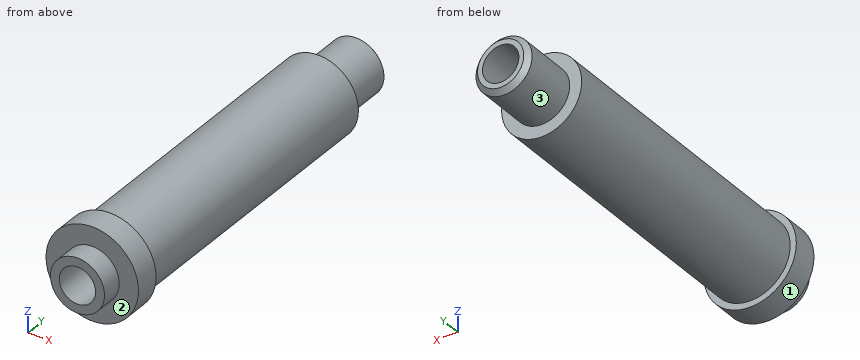
Autodesk Inventor part; units mm, degrees
ref_plane "YZ Plane" through (0, 0, 0) normal (1, 0, 0) x (0, 1, 0)
ref_plane "XZ Plane" through (0, 0, 0) normal (0, 1, 0) x (-1, 0, 0)
ref_plane "XY Plane" through (0, 0, 0) normal (0, 0, 1) x (1, 0, 0)
sketch "Sketch1" plane through (0, 0, 0) normal (0, 1, 0) x (-1, 0, 0)
  circle A0 centre (0, 0) radius 4.699
  dimension "d0" = 9.398
extrude "Extrusion1" add sketch "Sketch1" along normal blind 4.826
sketch "Sketch2" plane through (0, 0, 0) normal (0, -1, 0) x (1, 0, 0)
  circle A0 centre (0, 0) radius 4.075
  dimension "d3" = 8.15
extrude "Extrusion2" add sketch "Sketch2" against normal blind 35.866
sketch "Sketch3" plane through (0, 0, 0) normal (0, -1, 0) x (1, 0, 0)
  circle A0 centre (0, 0) radius 4.699
  circle A1 centre (0, 0) radius 2.75
  dimension "d18" = 5.5
extrude "Extrusion3" cut sketch "Sketch3" against normal blind 2.2
sketch "Sketch5" plane through (0, 0, 0) normal (0, -1, 0) x (1, 0, 0)
  circle A0 centre (0, 0) radius 2.75
hole "Hole2" at (0, 0, 0) direction (0, 1, 0) diameter 3.7 end through all
sketch "Sketch6" plane through (0, 35.866, 0) normal (0, 1, 0) x (1, 0, 0)
  circle A0 centre (0, 0) radius 1.85
  circle A1 centre (0, 0) radius 2.85
  dimension "d29" = 5.7
extrude "Extrusion4" add sketch "Sketch6" along normal blind 6.1
chamfer "Chamfer3" distance 0.5 angle 45 1 edges at (-2.85, 41.966, 0)
properties part number "Hour shaft test 7"
Geometry check sheet. Reference: the model listing, model coordinates, mm. Face numbers are marked on the shaded views. A direction names the side the tool comes from. Round coordinates to 2 decimals unless told otherwise and drop trailing zeros. Order: outer loops, then holes, each group sorted by start corner. A loop starts at its lowest first (then second) coordinate and runs counter-clockwise, first axis right, second up. Notation, with made-up numbers: (51.25, 89) - (79.25, 89) arc R18 ccw to (79.25, 111) - close; hole circle Ø8 at (-30, -16.75). An arc over 180 degrees is marked (long way). Use a Markdown table: item, result. Add a question column.
(1) Sectioned sample at A-A, the plane x = 0. Enter the section's corners in (y, z) (3 decimals), and give its area (3 significant figures).
(2) Sectioned sample at B-B, the plane z = 0. Enter the section's corners in (x, y) (3 decimals).
(3) Tool access check on the marked faces 1, 2 and 3. Record the directions out of +Z, -Z, +X, -X, +Y, -Y that give a thin tool (end or side, any length) a straight path to the whole face; none if there is none.
(4) Sectioned sample at D-D, the plane x = -3.5. Enter the section's corners in (y, z).
(5) Material ranges on line 1 along Z through (x, y) = (0, 40.5); line 2 along Z through (x, y) = (0, 13.5) (3 decimals), recorded low to high. Write a range as [from, to].
(6) Sectioned sample at C-C, the plane y = 21.5. Enter the section's corners in (x, z) (3 decimals), and give its area (3 significant figures).
(7) Depth check by flat-ended pin: pin 1 (1 mm diameter, centred on x = -3, z = -2.5, fed in from -Y); pin 2 (5 mm diameter, centred on x = 0, y = 33, fed in from +Z) (3 decimals); pin 3 (4 mm diameter, centred on x = 3.5, y = 27.5, fed in from -Z). Enter the tip coordinate at first touch or a pass-through.
Answers below:
| question | item | result |
|---|---|---|
| 1 | outline | (0, -2.75) - (2.2, -2.75) - (2.2, -4.699) - (4.826, -4.699) - (4.826, -4.075) - (35.866, -4.075) - (35.866, -2.85) - (41.466, -2.85) - (41.966, -2.35) - (41.966, -1.85) - (0, -1.85) - close; (0, 1.85) - (41.966, 1.85) - (41.966, 2.35) - (41.466, 2.85) - (35.866, 2.85) - (35.866, 4.075) - (4.826, 4.075) - (4.826, 4.699) - (2.2, 4.699) - (2.2, 2.75) - (0, 2.75) - close |
| 1 | area | 169 mm² |
| 2 | outline | (-4.699, 2.2) - (-2.75, 2.2) - (-2.75, 0) - (-1.85, 0) - (-1.85, 41.966) - (-2.35, 41.966) - (-2.85, 41.466) - (-2.85, 35.866) - (-4.075, 35.866) - (-4.075, 4.826) - (-4.699, 4.826) - close; (1.85, 0) - (2.75, 0) - (2.75, 2.2) - (4.699, 2.2) - (4.699, 4.826) - (4.075, 4.826) - (4.075, 35.866) - (2.85, 35.866) - (2.85, 41.466) - (2.35, 41.966) - (1.85, 41.966) - close |
| 3 | face 1 | +Y, -Y |
| 3 | face 2 | -Y |
| 3 | face 3 | +Y |
| 4 | outline | (2.2, -3.14) - (4.83, -3.14) - (4.83, -2.09) - (35.87, -2.09) - (35.87, 2.09) - (4.83, 2.09) - (4.83, 3.14) - (2.2, 3.14) - close |
| 5 | line 1 | [-2.85, -1.85], [1.85, 2.85] |
| 5 | line 2 | [-4.075, -1.85], [1.85, 4.075] |
| 6 | outline | circle Ø8.15 at (0, 0); hole circle Ø3.7 at (0, 0) |
| 6 | area | 41.4 mm² |
| 7 | pin 1 | y = 2.2 |
| 7 | pin 2 | z = 4.075 |
| 7 | pin 3 | z = -3.79 |
